Source: CAD feature listing. Evaluate the final solid. Frame: model axes, mm. Round coordinates to 2 decimals unless told otherwise and drop trailing zeros. Loops run counter-clockwise (first coordinate to the right, second up) from the corner with the lowest first, then second, coordinate; pieces in that order, holes last. Notation, with made-up numbers: (72.25, 64.5) -> (80.25, 64.5) arc R27 ccw to (80.25, 102.5) -> close; hole circle Ø8 at (-4, -34.5). An arc over 180 degrees is marked (long way). Put each result on its own line as item: value. Start each with the question number.
1. Material intervals for L1, parallel to X at y = 11.5, z = 30.5; L2, parallel to Z at x = 21.5, y = 7.25; L3, parallel to Z at x = -1.5, y = 1.5, sorted ascending.
2. Cut plane A-A (x = 0). Return the cut outline in (y, z), then the cut area to 3 significant figures.
3. Contact query for flat-ended pins moving along their axis: pin 1 (4 mm diameter, centred on x = 12.5, y = 9.5, fed in from -Z); pin 2 (8 mm diameter, centred on y = 7.5, z = 3, fed in from -X); pin 3 (5 mm diameter, centred on x = 11, y = 7, fed in from -Z). Output: stop coordinate, or through.
4. Cut plane D-D (y = 1.75). Return the cut outline in (x, z).
5. Cut plane C-C (y = 10). Return the cut outline in (x, z), then the cut area to 3 significant figures.
6. Cut plane B-B (z = 0). Return the cut outline in (x, y).
```python
from build123d import *

# Parameters (mm, degrees)
SKETCH2_R           = 110
BOSS_EXTRUDE1_DEPTH = 50
CHAMFER1_SIZE       = 15
SCALE1_SCALE        = 0.333333333


with BuildPart() as part:
    # Sketch2 → Boss-Extrude1 (new body)
    with BuildSketch(Plane(origin=(0, 0, 0), x_dir=(1, 0, 0), z_dir=(0, 1, 0))):
        with Locations(Location((0, 0, 0), (0, 0, 270))):
            Circle(SKETCH2_R)
    extrude(amount=BOSS_EXTRUDE1_DEPTH)

    # Chamfer1
    chamfer1_edges = [part.edges().sort_by_distance(p)[0] for p in [
        (0, 0, -110),
        (0, 50, -110),
    ]]
    chamfer(chamfer1_edges, length=CHAMFER1_SIZE)


with BuildPart() as part_1:
    # Scale1: scaled about (0, 0, 0)
    add(part.part.scale(SCALE1_SCALE))


solid = part_1.part
```
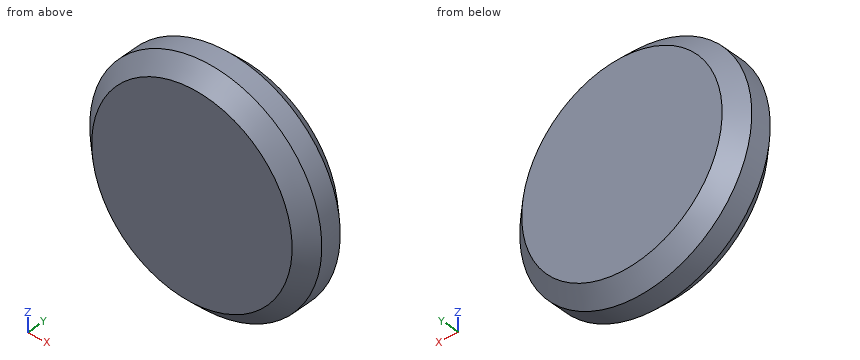
Solution:
1. L1: x = -20.35 to 20.35
1. L2: z = -29.7 to 29.7
1. L3: z = -33.13 to 33.13
2. outline: (0, -31.67) -> (5, -36.67) -> (11.67, -36.67) -> (16.67, -31.67) -> (16.67, 31.67) -> (11.67, 36.67) -> (5, 36.67) -> (0, 31.67) -> close
2. area: 1,170 mm^2
3. pin 1: stops at z = -35.13
3. pin 2: stops at x = -36.67
3. pin 3: stops at z = -35.67
4. outline: circle Ø66.83 at (0, 0)
5. outline: circle Ø73.33 at (0, 0)
5. area: 4,220 mm^2
6. outline: (-36.67, 5) -> (-31.67, 0) -> (31.67, 0) -> (36.67, 5) -> (36.67, 11.67) -> (31.67, 16.67) -> (-31.67, 16.67) -> (-36.67, 11.67) -> close
